Model file for the job. Use its own axes, mm. A direction names the side the tool comes from. Coordinates: 2 decimals unless noted, no trailing zeros. Loops run counter-clockwise (first coordinate to the right, second up) from the corner with the lowest first, then second, coordinate; pieces in that order, holes last.
Autodesk Fusion 360 part; units mm, degrees
sketch "Skizze1" plane through (0, 0, 0) normal (0, 0, 1) x (1, 0, 0)
  line L0 (0, 0) -> (8.2, 0)
  line L1 (8.2, 0) -> (8.2, 5)
  line L2 (8.2, 5) -> (0, 5)
  line L3 (0, 5) -> (0, 0)
  dimension "d1" = 8.2
  dimension "d2" = 5
extrude "Extrusion1" add sketch "Skizze1" along normal blind 8.2
sketch "Skizze2" plane through (0, 0, 8.2) normal (0, 0, 1) x (-1, 0, 0)
  line L0 (0, -5) -> (0, 0)
  line L1 (0, 0) -> (-8.2, 0)
  line L2 (-8.2, 0) -> (-8.2, -5)
  line L3 (-8.2, -5) -> (0, -5)
  circle A0 centre (-4.1, -2.5) radius 3
  dimension "d5" = 6
  dimension "d6" = 2.5
  dimension "d38" = 4.1
extrude "Extrusion2" add sketch "Skizze2" along normal blind 0.5 contours L3 A0 | L1 L3 A0 | L1 A0
sketch "Skizze3" plane through (0, 0, 8.7) normal (0, 0, 1) x (-1, 0, 0)
  circle A0 centre (-4.1, -2.5) radius 3
  circle A1 centre (-4.1, -2.5) radius 2.375
  dimension "d9" = 4.75
extrude "Extrusion3" add sketch "Skizze3" along normal blind 5.5 contours A1
sketch "Skizze4" plane through (0, 0, 14.2) normal (0, 0, 1) x (-1, 0, 0)
  circle A0 centre (-4.1, -2.5) radius 2.375
  circle A1 centre (-4.1, -2.5) radius 1.25
  dimension "d12" = 2.5
sketch "Skizze5" plane through (0, 0, 0) normal (0, 0, -1) x (1, 0, 0)
  line L0 (0, 0) -> (0, -5)
  line L1 (0, -5) -> (8.2, -5)
  line L2 (8.2, -5) -> (8.2, 0)
  line L3 (8.2, 0) -> (0, 0)
  circle A0 centre (4.1, -2.5) radius 1
  circle A1 centre (6.6, -2.5) radius 1
  circle A2 centre (1.6, -2.5) radius 1
  dimension "d17" = 2
  dimension "d18" = 2.5
  dimension "d21" = 2.5
  dimension "d22" = 0
  dimension "d25" = -2.5
  dimension "d26" = 0
  dimension "d39" = 4.1
extrude "Extrusion5" add sketch "Skizze5" along normal blind 5 contours A0 | A1 | A2
sketch "Skizze6" plane through (0, 0, 8.7) normal (0, 0, 1) x (-1, 0, 0)
  circle A0 centre (-4.1, -2.5) radius 2.375
  circle A1 centre (-4.1, -2.5) radius 3
  line L0 (-7.3757, -3.7328) -> (-4.6702, -5.9532)
  line L1 (-4.6702, -5.9532) -> (-1.3945, -4.7204)
  line L2 (-1.3945, -4.7204) -> (-0.8243, -1.2672)
  line L3 (-0.8243, -1.2672) -> (-3.5298, 0.9532)
  line L4 (-3.5298, 0.9532) -> (-6.8055, -0.2796)
  line L5 (-6.8055, -0.2796) -> (-7.3757, -3.7328)
  point P0 (-4.1, -2.5)
  dimension "d29" = 3.5
extrude "Extrusion6" add sketch "Skizze6" along normal blind 1.5 contours A1 | L0 L1 L2 L3 L4 L5
ref_plane "Arbeitsebene1" through (4.1, 2.5, 12.2) normal (0, 0, 1) x (-1, 0, 0)
sketch "Skizze8" plane through (4.1, 2.5, 12.2) normal (0, 0, 1) x (1, 0, 0)
  line L0 (-1.1793, 3.2572) -> (-3.4105, 0.6073)
  line L1 (-3.4105, 0.6073) -> (-2.2311, -2.6499)
  line L2 (-2.2311, -2.6499) -> (1.1793, -3.2572)
  line L3 (1.1793, -3.2572) -> (3.4105, -0.6073)
  line L4 (3.4105, -0.6073) -> (2.2311, 2.6499)
  line L5 (2.2311, 2.6499) -> (-1.1793, 3.2572)
  dimension "d40" = 3
extrude "Extrusion9" add sketch "Skizze8" along normal blind 1.5
sketch "Skizze9" plane through (0, 0, 14.2) normal (0, 0, 1) x (-1, 0, 0)
  circle A0 centre (-4.1, -2.5) radius 2.375
  circle A1 centre (-4.1, -2.5) radius 1
  dimension "d43" = 2
extrude "Extrusion10" add sketch "Skizze9" along normal blind 10 draft 2.5 contours A1
fillet "Abrundung2" radius 1 1 edges at (5.4394, 1.9805, 24.2)
Q1. Which spindle directions (+Z, -Z, +X, -X, +Y, -Y) get a long thin tool onto all of the face, cutting with end or side? Do faces 1 (the flat face through (0.7, 2.5, 8.2)), 2 (the flat face through (4.65, 5.45, 12.94)), 3 (the flat face through (1.27, 1.5, 12.94)), 4 (the flat face through (7.087, 1.982, 9.439)), 5 (the flat face through (3, 0, 12.2)). Say none if no direction does.
Answers:
face 1: -X
face 2: +Z, +X, +Y
face 3: +Z, -X, -Y
face 4: +X, -Y
face 5: none
Q2. Flat gauge pins, fed straight in: P1, Ø1.5, axis at y = 1, z = 10.5, coming from the -X side; P2, Ø2, axis at y = 0.5, z = 19.5, coming from the +X side; P3, Ø1.4, axis at x = 3.5, y = 3.5, coming from the +Z side. Where does each tip first touch, or does it go through?
Answers:
P1: stops at x = 0.82
P2: stops at x = 4.82
P3: stops at z = 24.2
Q3. Slice it at C-C (z = 2). List the corners of the cut face in (x, y).
Answers:
outline: (0, 0) - (8.2, 0) - (8.2, 5) - (0, 5) - close
Q4. Slice it at B-B (z = -2). List the corners of the cut face in (x, y), and give its area (3 significant figures).
Answers:
outline: circle Ø2 at (1.6, 2.5); circle Ø2 at (4.1, 2.5); circle Ø2 at (6.6, 2.5)
area: 9.42 mm2
Q5. Mould opens along Z. For faces 6 (the flat face through (7, 2, -5)), 7 (the cylindrical face through (1.24, 3.4, 8.45)), 8 (the flat face through (3.055, 5.345, 9.439)) say: +Z half, -Z half, draft (parallel to the pull), parting line (faces both ways), or undercut.
Answers:
face 6: -Z half
face 7: undercut
face 8: draft
Q6. Drill centre lines: line 1 (Z direction, x = 2, y = 4.25); line 2 (Z direction, x = 6.5, y = 4.5); line 3 (Z direction, x = 7.75, y = 4.5). Where is each one in solid material? Low to high.
Answers:
line 1: z = 0 to 10.2, 12.2 to 13.7
line 2: z = 0 to 8.2, 12.2 to 13.7
line 3: z = 0 to 8.2
Q7. Slice it at A-A (z = 12.75). List the corners of the cut face in (x, y).
Answers:
outline: (0.69, 3.11) - (1.87, -0.15) - (5.28, -0.76) - (7.51, 1.89) - (6.33, 5.15) - (2.92, 5.76) - close
